from build123d import *

# Parameters (mm, degrees)
SKETCH1_W           = 21.1836
SKETCH1_H           = 21.1836
BOSS_EXTRUDE1_DEPTH = 1219.2
SKETCH2_R           = 8.001
CUT_EXTRUDE1_DEPTH  = 1219.2


with BuildPart() as part:
    # Sketch1 → Boss-Extrude1 (new body)
    with BuildSketch(Plane.XY):
        with BuildLine():
            Line((-9.525, -12.7), (9.525, -12.7))
            ThreePointArc((9.525, -12.7), (11.77006403, -11.77006403), (12.7, -9.525))
            Line((12.7, -9.525), (12.7, 9.525))
            ThreePointArc((12.7, 9.525), (11.77006403, 11.77006403), (9.525, 12.7))
            Line((9.525, 12.7), (-9.525, 12.7))
            ThreePointArc((-9.525, 12.7), (-11.77006403, 11.77006403), (-12.7, 9.525))
            Line((-12.7, 9.525), (-12.7, -9.525))
            ThreePointArc((-12.7, -9.525), (-11.77006403, -11.77006403), (-9.525, -12.7))
        make_face()
        Rectangle(SKETCH1_W, SKETCH1_H, mode=Mode.SUBTRACT)
    extrude(amount=BOSS_EXTRUDE1_DEPTH)

    # Sketch2 → Cut-Extrude1 (cut)
    with BuildSketch(Plane(origin=(0, 12.7, 0), x_dir=(1, 0, 0), z_dir=(0, 1, 0))):
        with Locations(Location((0, -1193.8, 0), (0, 0, 270))):
            Circle(SKETCH2_R)
        with Locations(Location((0, -1143, 0), (0, 0, 270))):
            Circle(SKETCH2_R)
    extrude(amount=-CUT_EXTRUDE1_DEPTH, mode=Mode.SUBTRACT)


solid = part.part
Here's how the part is built. I have some questions about the finished solid (model axes, mm). A direction names the side the tool comes from. Round coordinates to 2 decimals unless told otherwise and drop trailing zeros. Write each loop counter-clockwise with the first axis right and the second up, starting at its lowest first coordinate (ties: lowest second). Pieces come first, ordered by that corner, then holes. Notation, with made-up numbers: (30, 14.25) -> (75, 14.25) arc R22 ccw to (75, 34.25) -> close; hole circle Ø6 at (-29.5, 87). An arc over 180 degrees is marked (long way). One line per item, written item: value.
1) We'd pull the mould along Y, two halves only. Please class faces 3 (the face through (-10.592, 0, 601)), 4 (the face through (-12.7, 0, 601)), 5 (the face through (0, 12.7, 601)): released by +Y, released by -Y, zero draft, split by the parting line, or undercut.
Filled sheet:
face 3: undercut
face 4: zero draft
face 5: released by +Y
2) If I drill on line 1 (X direction, y = 3.5, z = 654.5); line 2 (X direction, y = 11.5, z = 1143), over which ranges is the centre line in solid material (lowest first)? Write a range as [from, to].
Filled sheet:
line 1: x = [-12.7, -10.59], [10.59, 12.7]
line 2: x = [-12.01, -8], [8, 12.01]
3) I'm going to push a flat-ended pin straight in: pin 1 Ø5 at (x, y) = (3, -6.5) entering from -Z. Where does the tip first touch, or does it pass through?
Filled sheet:
pin 1: passes through
4) Suppose I cut it at B-B on x = 0. List the corners of the cut face in (y, z) for me, plus the area to 3 significant figures.
Filled sheet:
outline: (-12.7, 0) -> (-10.59, 0) -> (-10.59, 1135) -> (-12.7, 1135) -> close; (-12.7, 1151) -> (-10.59, 1151) -> (-10.59, 1185.8) -> (-12.7, 1185.8) -> close; (-12.7, 1201.8) -> (-10.59, 1201.8) -> (-10.59, 1219.2) -> (-12.7, 1219.2) -> close; (10.59, 0) -> (12.7, 0) -> (12.7, 1135) -> (10.59, 1135) -> close; (10.59, 1151) -> (12.7, 1151) -> (12.7, 1185.8) -> (10.59, 1185.8) -> close; (10.59, 1201.8) -> (12.7, 1201.8) -> (12.7, 1219.2) -> (10.59, 1219.2) -> close
area: 5,010 mm2
5) Suppose I cut it at C-C on y = -4.25. List the corners of the cut face in (x, z) for me.
Filled sheet:
outline: (-12.7, 0) -> (-10.59, 0) -> (-10.59, 1219.2) -> (-12.7, 1219.2) -> close; (10.59, 0) -> (12.7, 0) -> (12.7, 1219.2) -> (10.59, 1219.2) -> close
6) Suppose I cut it at A-A on z = 172.5. List the corners of the cut face in (x, y) for me (3 decimals), plus the area to 3 significant figures.
Filled sheet:
outline: (-12.7, -9.525) arc R3.175 ccw to (-9.525, -12.7) -> (9.525, -12.7) arc R3.175 ccw to (12.7, -9.525) -> (12.7, 9.525) arc R3.175 ccw to (9.525, 12.7) -> (-9.525, 12.7) arc R3.175 ccw to (-12.7, 9.525) -> close; hole (-10.592, -10.592) -> (10.592, -10.592) -> (10.592, 10.592) -> (-10.592, 10.592) -> close
area: 188 mm2
7) For faces 1 (the face through (0, -10.592, 601)), 2 (the face through (12.7, 0, 601)), which set-ups out of +Z, -Z, +X, -X, +Y, -Y let a thin tool reach every point of the face, with its end or its side?
Filled sheet:
face 1: +Z, -Z
face 2: +Z, -Z, +X, +Y, -Y
